For this review, use the dimensioned drawing (mm, ordinates from the lowest corner) and the shaded views. A direction names the side the tool comes from. Give positions to 0.01 mm unless a question says otherwise; leave off trailing zeros. Loops run counter-clockwise (first coordinate to the right, second up) from the corner with the lowest first, then second, coordinate; pieces in that order, holes last. Notation, with made-up numbers: M 64.5,1 L 87.5,1 A34 ccw 87.5,37 Z; hole C 2,-16 d10. An arc over 180 degrees is marked long. Use one line per item in the form item = value. Start each with the question number.
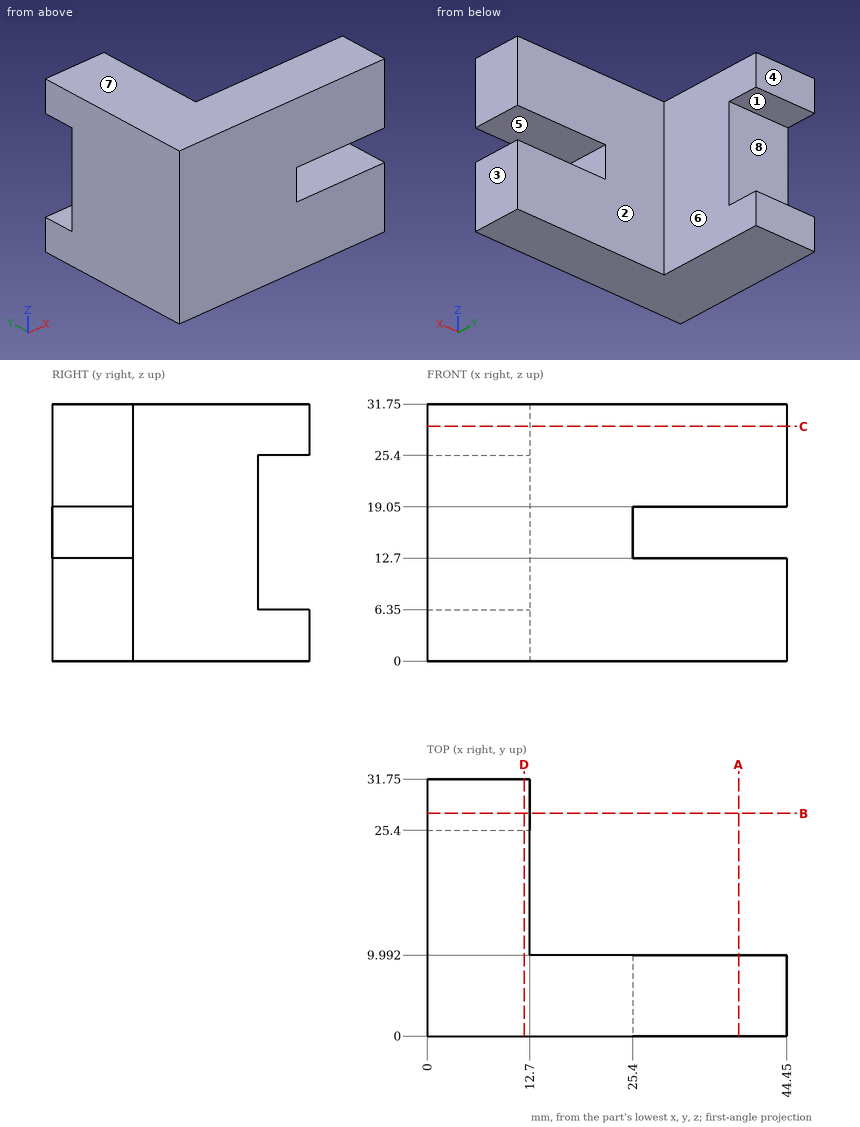
Q1. Take a section at B-B on y = 27.5. Give the boundary of the cut face in (x, z).
Q2. The part is to be moulded in two halves that separate along Z. For the marked faces 6, 7 and 8, say which applies: pulls with the +Z half, pulls with the -Z half, needs draft (parallel to the pull), parting line crosses it, or undercut.
Q3. Wall thickness on probe 1 along Z at (x, y) = (11, 27.5); probe 2 along Z at (x, y) = (41, 3); probe 3 along X at (y, z) = (19.5, 4): over which ranges is each line inside the solid? List them lowest first.
Q4. Take a section at A-A on x = 38.5. Give the boundary of the cut face in (y, z).
Q5. For the marked faces 1, 2, 3, 4 and 5, list the 3-axis set-ups (+Z, -Z, +X, -X, +Y, -Y) from which the entire face can be reached by the end or side of a thin tool; tool diameter is ignored.
Q6. Clearance check with flat-ended pins moving along their axes: pin 1 Ø4 at (x, z) = (40, 13) entering from +Y; pin 2 Ø1.9 at (y, z) = (7.5, 15.5) entering from +X; pin 3 Ø8 at (x, y) = (23, 15) entering from -Z; pin 4 Ø5 at (y, z) = (21.5, 11.5) entering from +X. State where each tip first meets the part, or that it passes through.
Q7. Take a section at C-C on z = 29. Give the boundary of the cut face in (x, y).
Q8. Take a section at D-D on x = 12. Give the boundary of the cut face in (y, z).
Response values:
q1.outline = M 0,0 L 12.7,0 L 12.7,6.35 L 0,6.35 Z; M 0,25.4 L 12.7,25.4 L 12.7,31.75 L 0,31.75 Z
q2.face_6 = needs draft
q2.face_7 = pulls with the +Z half
q2.face_8 = undercut
q3.probe_1 = 0 to 6.35, 25.4 to 31.75
q3.probe_2 = 0 to 12.7, 19.05 to 31.75
q3.probe_3 = 0 to 12.7
q4.outline = M 0,0 L 9.99,0 L 9.99,12.7 L 0,12.7 Z; M 0,19.05 L 9.99,19.05 L 9.99,31.75 L 0,31.75 Z
q5.face_1 = +X, -X, +Y
q5.face_2 = +Z, -Z, +X, +Y
q5.face_3 = +Z, -Z, +X, +Y, -Y
q5.face_4 = +Z, -Z, +X, -X, +Y
q5.face_5 = +X, +Y, -Y
q6.pin_1 = 9.99
q6.pin_2 = 25.4
q6.pin_3 = through
q6.pin_4 = 12.7
q7.outline = M 0,0 L 44.45,0 L 44.45,9.99 L 12.7,9.99 L 12.7,31.75 L 0,31.75 Z
q8.outline = M 0,0 L 31.75,0 L 31.75,6.35 L 25.4,6.35 L 25.4,25.4 L 31.75,25.4 L 31.75,31.75 L 0,31.75 Z
